Check sheet for the modelled part. Datum: model origin and axes. Units: mm. A direction names the side the tool comes from. Give positions to 0.01 mm unless a question says otherwise; leave off trailing zeros. Write each loop counter-clockwise with the first axis right and the second up, starting at its lowest first coordinate (ties: lowest second). Pieces come first, ordered by that corner, then holes. Notation, with made-up numbers: M 58.25,-12 L 64.25,-12 A15 ccw 64.25,-3 Z; hole C 25.25,26.25 d5. An arc over 180 degrees is marked long. Write item = value, one per line. Start each with the question number.
1) Sectioned sample at A-A, the plane z = 6. Record the cut outline in (x, y).
2) Gauge pin test, flat ends, axial feed: pin 1 (5.5 mm diameter, centred on x = -2.5, y = 17, fed in from +Z); pin 2 (3.5 mm diameter, centred on x = -2, y = -14.5, fed in from +Z). Record the tip position at first contact, or that the pin passes through.
3) Draft check along X on faces 3 (the face through (6.5, -29.5, 5.9)), 4 (the face through (0, -11, 5.2)), 5 (the face through (-1.774, -17.783, 2.564)), 6 (the face through (0, 30, 6)). Enter one of: pulls with the +X half, pulls with the -X half, needs draft (parallel to the pull), parting line crosses it, or undercut.
4) Scan lines: L1, parallel to Y at x = -2, z = 9.25; L2, parallel to Y at x = 0, z = 3.75; L3, parallel to Y at x = -1.25, z = 7.75. Record each from-to range of solid material in increasing order.
5) Sectioned sample at C-C, the plane x = 0. Record the cut outline in (y, z), then the cut area to 3 significant figures.
6) Set-up check for faces 1 (the face through (-7, 0, 3)), 2 (the face through (0, 11, 5.2)): record each of +Z, -Z, +X, -X, +Y, -Y from which the full face is reachable in a straight line by a thin tool's end or side.
7) Sectioned sample at D-D, the plane z = 1.75. Record the cut outline in (x, y).
8) Sectioned sample at B-B, the plane y = 15. Record the cut outline in (x, z), then the cut area to 3 significant figures.
from build123d import *

# Parameters (mm, degrees)
SKETCH_1_W                   = 14
SKETCH_1_H                   = 60
EXTRUDE_1_DEPTH              = 12
HOLE_WIZARD_M6_1_D           = 6.6
HOLE_WIZARD_M6_1_CBORE_D     = 11
HOLE_WIZARD_M6_1_CBORE_DEPTH = 6.8
CHAMFER_1_SIZE               = 1
HOLE_WIZARD_M5_1_D           = 4.2


with BuildPart() as part:
    # 草图1 → 凸台-拉伸1 (new body)
    with BuildSketch(Plane.XY):
        Rectangle(SKETCH_1_W, SKETCH_1_H)
    extrude(amount=EXTRUDE_1_DEPTH)

    # M6 六角圆柱头螺钉的柱形沉头孔1 (through all)
    with Locations(Plane.XY.offset(12)):
        with Locations((0, 15)):
            hole_wizard_m6_1 = CounterBoreHole(HOLE_WIZARD_M6_1_D / 2, HOLE_WIZARD_M6_1_CBORE_D / 2, HOLE_WIZARD_M6_1_CBORE_DEPTH)

    # 镜向1: M6 六角圆柱头螺钉的柱形沉头孔1 across plane
    add(hole_wizard_m6_1.mirror(Plane.ZX), mode=Mode.SUBTRACT)

    # 倒角1
    chamfer_1_edges = [part.edges().sort_by_distance(p)[0] for p in [
        (7, -30, 6),
        (-7, -30, 6),
        (-7, 30, 6),
        (7, 30, 6),
    ]]
    chamfer(chamfer_1_edges, length=CHAMFER_1_SIZE)

    # M5 螺纹孔1 (through all)
    with Locations(Plane(origin=(7, 0, 0), x_dir=(0, 0, -1), z_dir=(1, 0, 0))):
        with Locations((-6, 0)):
            Hole(HOLE_WIZARD_M5_1_D / 2)


solid = part.part
Data:
q1.outline = M -7,-29 L -6,-30 L 6,-30 L 7,-29 L 7,-2.1 L -7,-2.1 Z; M -7,2.1 L 7,2.1 L 7,29 L 6,30 L -6,30 L -7,29 Z; hole C 0,-15 d11; hole C 0,15 d11
q2.pin_1 = 12
q2.pin_2 = 5.2
q3.face_3 = pulls with the +X half
q3.face_4 = undercut
q3.face_5 = undercut
q3.face_6 = needs draft
q4.L1 = -30 to -20.12, -9.88 to 9.88, 20.12 to 30
q4.L2 = -30 to -18.3, -11.7 to 11.7, 18.3 to 30
q4.L3 = -30 to -20.36, -9.64 to -1.16, 1.16 to 9.64, 20.36 to 30
q5.outline = M -30,0 L -18.3,0 L -18.3,5.2 L -20.5,5.2 L -20.5,12 L -30,12 Z; M -11.7,0 L 11.7,0 L 11.7,5.2 L 9.5,5.2 L 9.5,12 L -9.5,12 L -9.5,5.2 L -11.7,5.2 Z; M 18.3,0 L 30,0 L 30,12 L 20.5,12 L 20.5,5.2 L 18.3,5.2 Z; hole C 0,6 d4.2
q5.area = 488 mm2
q6.face_1 = +Z, -Z, -X, +Y, -Y
q6.face_2 = +Z
q7.outline = M -7,-29 L -6,-30 L 6,-30 L 7,-29 L 7,29 L 6,30 L -6,30 L -7,29 Z; hole C 0,-15 d6.6; hole C 0,15 d6.6
q8.outline = M -7,0 L -3.3,0 L -3.3,5.2 L -5.5,5.2 L -5.5,12 L -7,12 Z; M 3.3,0 L 7,0 L 7,12 L 5.5,12 L 5.5,5.2 L 3.3,5.2 Z
q8.area = 58.9 mm2
